Autodesk Inventor part; units mm, degrees
ref_plane "YZ Plane" through (0, 0, 0) normal (1, 0, 0) x (0, 1, 0)
ref_plane "XZ Plane" through (0, 0, 0) normal (0, 1, 0) x (-1, 0, 0)
ref_plane "XY Plane" through (0, 0, 0) normal (0, 0, 1) x (1, 0, 0)
sketch "Sketch1" plane through (0, 0, 0) normal (0, 1, 0) x (-1, 0, 0)
  circle A0 centre (-18.3582, -14.9546) radius 2.1844
  circle A1 centre (-26.8299, -5.4931) radius 2.1844
  circle A2 centre (34.045, -0.5216) radius 2.1844
  circle A3 centre (19.4876, 18.9331) radius 2.1844
  circle A4 centre (11.0156, 28.3943) radius 2.1844
  circle A5 centre (-18.3582, -14.9546) radius 6.35
  circle A6 centre (19.4876, 18.9331) radius 6.35
  circle A7 centre (34.045, -0.5216) radius 6.35
  circle A8 centre (11.0156, 28.3943) radius 6.35
  circle A9 centre (-26.8299, -5.4931) radius 6.35
  line L0 (6.7797, 33.125) -> (-31.0658, -0.7624)
  line L1 (15.7462, 32.6303) -> (24.2182, 23.1691)
  line L2 (-23.0889, -19.1904) -> (-31.5606, -9.729)
  line L3 (-16.672, -21.0766) -> (35.7311, -6.6437)
  line L4 (39.1292, 3.2827) -> (24.5718, 22.7374)
  point P0 (0, 0)
  dimension "d0" = 4.3688
  dimension "d1" = 4.3688
  dimension "d2" = 4.3688
  dimension "d3" = 12.7
  dimension "d4" = 12.7
  dimension "d5" = 12.7
extrude "Extrusion1" add sketch "Sketch1" along normal blind 1.5875
properties part number "stackBrace"
Geometry: final body of the model. Coordinates: model frame, mm. Round coordinates to 2 decimals unless told otherwise and drop trailing zeros. Loops run counter-clockwise (first coordinate to the right, second up) from the corner with the lowest first, then second, coordinate; pieces in that order, holes last. Notation, with made-up numbers: (23, 12) -> (42, 12) arc R10 cw to (42, 20) -> close; hole circle Ø3 at (44.25, 61). An arc over 180 degrees is marked (long way). Write each question's results on one line, items separated by ' | '.
Item 1: Cut plane B-B on y = 0.7. State how many separate pieces and enclosed holes the cut face has, and give its area (4 significant figures).
Answers below:
separate pieces: 1 | enclosed holes: 5 | area: 2,295 mm²
Item 2: Cut plane D-D on x = -26. Return the cut outline in (y, z), and give its area (3 significant figures).
Answers below:
outline: (0, -9.32) -> (1.59, -9.32) -> (1.59, 20.83) -> (0, 20.83) -> close | area: 47.9 mm²
Item 3: Pull-direction query (X, two-part tool) for faces 1 (the face through (-9.16, 0.78, -13.96)), 2 (the face through (-12.024, 0.783, 30.332)), 3 (the face through (33.174, 0.783, -5.213)); classes: pulls with the +X half, pulls with the -X half, needs draft (parallel to the pull), parting line crosses it, or undercut.
Answers below:
face 1: pulls with the -X half | face 2: undercut | face 3: pulls with the +X half
Item 4: Cut plane C-C on x = 27. Return the cut outline in (y, z), and give its area (3 significant figures).
Answers below:
outline: (0, -14.82) -> (1.59, -14.82) -> (1.59, -7.67) -> (0, -7.67) -> close; (0, -3.32) -> (1.59, -3.32) -> (1.59, 2.88) -> (0, 2.88) -> close | area: 21.2 mm²
Item 5: Line query: probe 1 along Z at (x, y) = (-36, 0.35); probe 2 along X at (y, z) = (0.6, 19.5); probe 3 along Z at (x, y) = (19, 0.2). Output: solid intervals per line, ascending. Write a range as [from, to].
Answers below:
probe 1: z = [-6.56, -1.5], [0.45, 7.46] | probe 2: x = [-26.99, -21.6], [-17.38, 8.44] | probe 3: z = [-21.27, -17.04], [-12.87, 10.04]
Item 6: Cut plane A-A on z = 20. Return the cut outline in (x, y).
Answers below:
outline: (-26.62, 0) -> (-21.39, 0) -> (-21.39, 1.59) -> (-26.62, 1.59) -> close; (-17.58, 0) -> (7.88, 0) -> (7.88, 1.59) -> (-17.58, 1.59) -> close
Item 7: Pin query (flat end, axial travel): pin 1 Ø3.5 at (x, z) = (18.36, -14.95) entering from -Y. Return the tip coordinate at first contact, or that it passes through.
Answers below:
pin 1: passes through
